Can you work these out from the drawing? Everything is in mm from the part's minimum corner. A direction names the side the tool comes from. Round coordinates to 2 decimals unless told otherwise and drop trailing zeros. Write each loop counter-clockwise with the first axis right and the second up, starting at its lowest first coordinate (ties: lowest second). Pieces come first, ordered by that corner, then holes. Notation, with made-up numbers: M 64.5,82.25 L 99.5,82.25 A20 ccw 99.5,107.25 Z; hole C 54,28 d11. An arc over 180 degrees is marked long. Answer in a Markdown table with one row per item. Add a question column.
(1) If we mould it in two halves opening along X, with no side actions, what happens to the marked faces 1, 2 and 3? For each: released by +X, released by -X, zero draft, split by the parting line, or undercut.
(2) Suppose I cut it at C-C, the plane y = 15.5. Write out the boundary of the cut face in (x, z), then the cut area to 3 significant figures.
(3) Suppose I cut it at A-A, the plane y = 6.25. Write out the boundary of the cut face in (x, z), then the cut area to 3 significant figures.
(4) I'm going to push flat-ended pins straight in: pin 1 (4 mm diameter, centred on y = 3.5, z = 8, fed in from -X); pin 2 (4 mm diameter, centred on x = 15.5, y = 4.5, fed in from +Z); pin 3 (8 mm diameter, centred on y = 8.5, z = 32, fed in from -X); pin 4 (2 mm diameter, centred on x = 46, y = 9, fed in from -Z). Where does each tip first touch, or does it pass through?
(5) Suppose I cut it at B-B, the plane z = 30. Write out the boundary of the cut face in (x, y).
(6) For the marked faces 4 and 5, which set-ups out of +Z, -Z, +X, -X, +Y, -Y let a thin tool reach every point of the face, with its end or its side?
(7) If I drill on probe 1 along X at (y, z) = (3, 30); probe 2 along X at (y, z) = (9, 35.5); probe 3 along Z at (x, y) = (39.5, 4.25), over which ranges is the centre line in solid material (lowest first)?
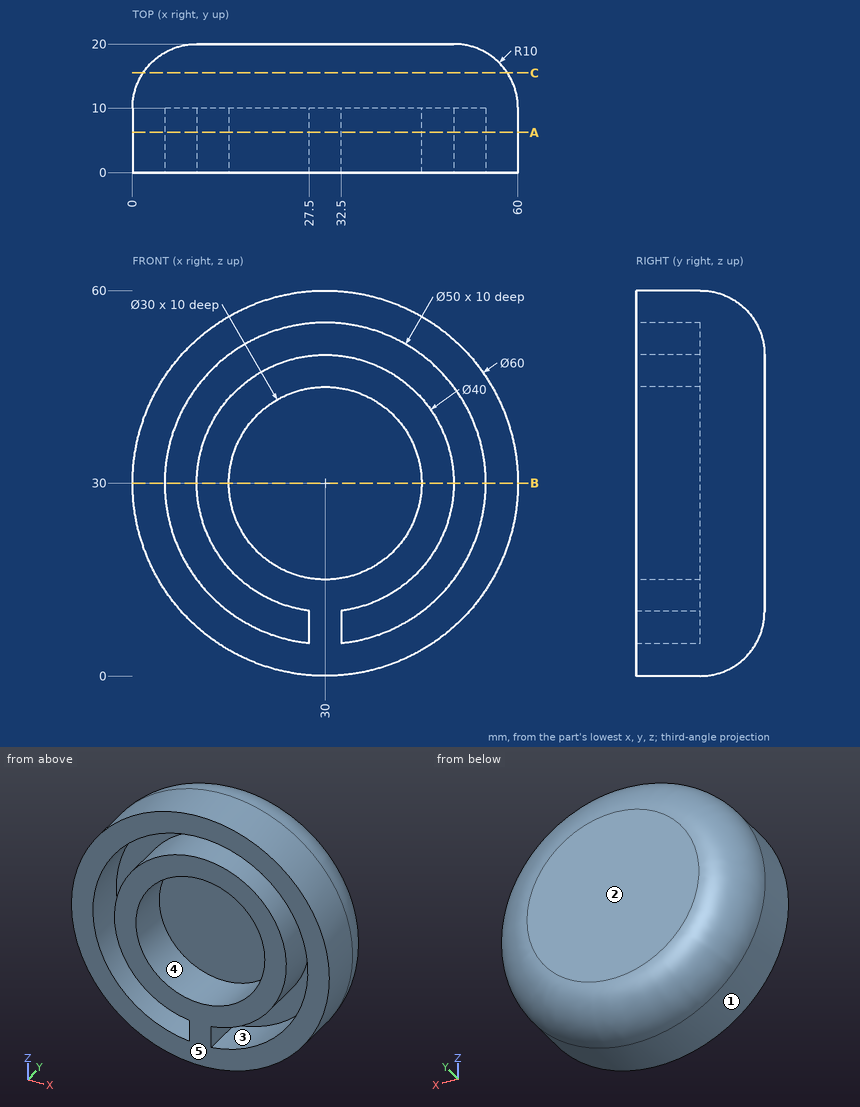
Calculated:
| question | item | result |
|---|---|---|
| 1 | face 1 | split by the parting line |
| 1 | face 2 | zero draft |
| 1 | face 3 | undercut |
| 2 | outline | C 30,30 d56.7 |
| 2 | area | 2,530 mm² |
| 3 | outline | C 30,30 d60; hole C 30,30 d30; hole M 27.5,5.13 L 27.5,10.16 A20 cw long 32.5,10.16 L 32.5,5.13 A25 ccw long Z |
| 3 | area | 1,440 mm² |
| 4 | pin 1 | x = 7.64 |
| 4 | pin 2 | z = 57.27 |
| 4 | pin 3 | x = 0 |
| 4 | pin 4 | z = 4.02 |
| 5 | outline | M 0,0 L 5,0 L 5,10 L 10,10 L 10,0 L 15,0 L 15,10 L 45,10 L 45,0 L 50,0 L 50,10 L 55,10 L 55,0 L 60,0 L 60,10 A10 ccw 50,20 L 10,20 A10 ccw 0,10 Z |
| 6 | face 4 | -Y |
| 6 | face 5 | +Z, -Z, +X, -X, -Y |
| 7 | probe 1 | 0 to 5, 10 to 15, 45 to 50, 55 to 60 |
| 7 | probe 2 | 0.51 to 5.61, 10.77 to 16.04, 43.96 to 49.23, 54.39 to 59.49 |
| 7 | probe 3 | 1.54 to 6.88, 12.4 to 18.39, 41.61 to 47.6, 53.12 to 58.46 |
